Here's the drawing with two shaded views (mm, measured from the low corner). I have some questions. A direction names the side the tool comes from. Give positions to 0.01 mm unless a question says otherwise; leave off trailing zeros. Write each loop counter-clockwise with the first axis right and the second up, starting at its lowest first coordinate (ties: lowest second). Pieces come first, ordered by that corner, then holes.
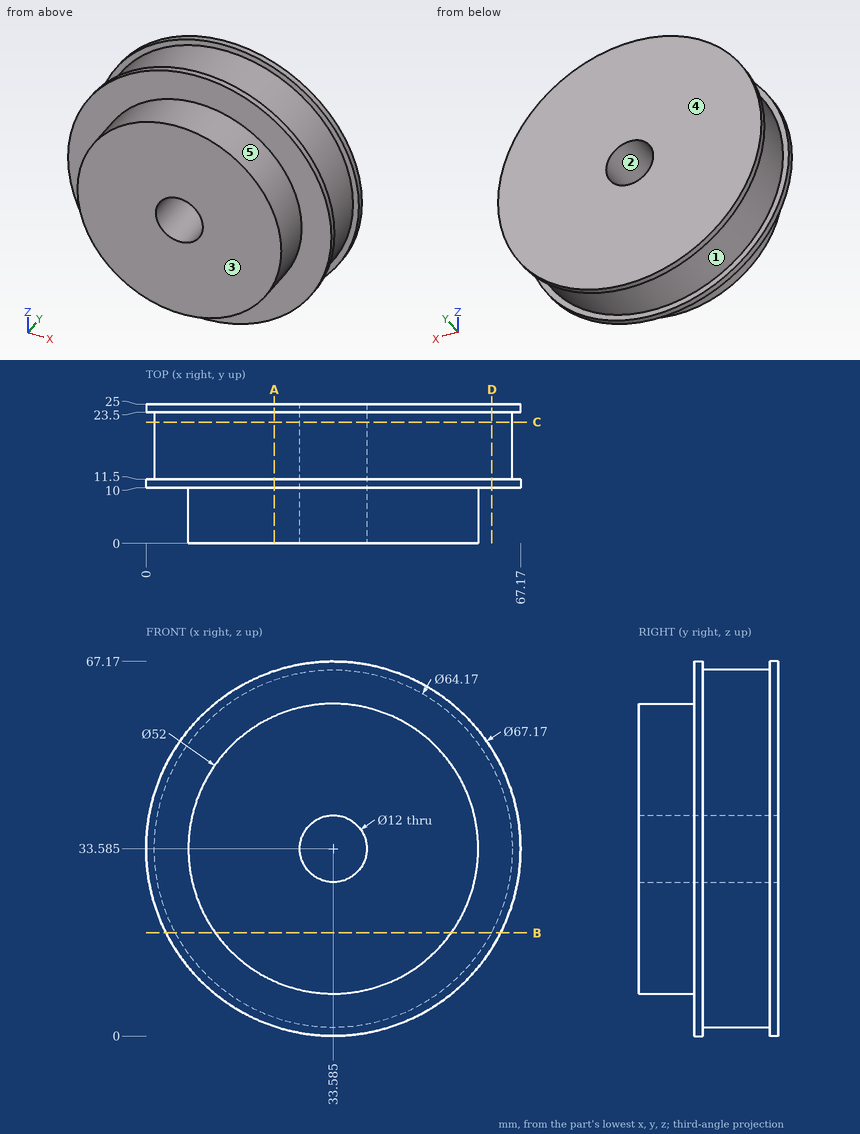
1) Please list where these lines run through material, in increasing order: L1, parallel to Y at x = 6.5, z = 52.5; L2, parallel to Z at x = 32, y = 11; L3, parallel to Y at x = 8, z = 23.
Values follow:
L1: y = 10 to 11.5, 23.5 to 25
L2: z = 0.04 to 27.8, 39.37 to 67.13
L3: y = 10 to 25
2) For pin 1 Ø8 at (y, z) = (12, 56) entering from -X; pin 2 Ø8 at (x, y) = (42, 4) entering from +Z; pin 3 Ø1.5 at (y, z) = (11.5, 8) entering from +X; pin 4 Ø5 at (x, z) = (8, 22) entering from -Y, each with a flat end and sliding along its axis, tell me the tip position at first contact or that it passes through.
Values follow:
pin 1: stops at x = 5.52
pin 2: stops at z = 59.21
pin 3: stops at x = 56.19
pin 4: stops at y = 0
3) If we mould it in two halves opening along X, with no side actions, what happens to the marked faces 1, 2 and 3? For each: +X half, -X half, draft (parallel to the pull), parting line (faces both ways), or undercut.
Values follow:
face 1: parting line
face 2: undercut
face 3: draft
4) For the marked faces 4 and 5, which set-ups out of +Z, -Z, +X, -X, +Y, -Y let a thin tool reach every point of the face, with its end or its side?
Values follow:
face 4: +Z, -Z, +X, -X, +Y
face 5: -Y
5) Suppose I cut it at C-C on y = 21.75. Write out the boundary of the cut face in (x, z) (3 decimals), plus the area to 3 significant figures.
Values follow:
outline: circle Ø64.17 at (33.585, 33.585); hole circle Ø12 at (33.585, 33.585)
area: 3,120 mm2
6) Suppose I cut it at D-D on x = 62. Write out the boundary of the cut face in (y, z), plus the area to 3 significant figures.
Values follow:
outline: (10, 15.68) - (11.5, 15.68) - (11.5, 18.68) - (23.5, 18.68) - (23.5, 15.68) - (25, 15.68) - (25, 51.49) - (23.5, 51.49) - (23.5, 48.49) - (11.5, 48.49) - (11.5, 51.49) - (10, 51.49) - close
area: 465 mm2
7) Suppose I cut it at A-A on x = 23. Write out the boundary of the cut face in (y, z).
Values follow:
outline: (0, 9.84) - (10, 9.84) - (10, 1.71) - (11.5, 1.71) - (11.5, 3.3) - (23.5, 3.3) - (23.5, 1.71) - (25, 1.71) - (25, 65.46) - (23.5, 65.46) - (23.5, 63.87) - (11.5, 63.87) - (11.5, 65.46) - (10, 65.46) - (10, 57.33) - (0, 57.33) - close
8) Suppose I cut it at B-B on z = 18.5. Write out the boundary of the cut face in (x, y).
Values follow:
outline: (3.58, 10) - (12.41, 10) - (12.41, 0) - (54.76, 0) - (54.76, 10) - (63.59, 10) - (63.59, 11.5) - (61.9, 11.5) - (61.9, 23.5) - (63.59, 23.5) - (63.59, 25) - (3.58, 25) - (3.58, 23.5) - (5.27, 23.5) - (5.27, 11.5) - (3.58, 11.5) - close
